Read the model definition and answer for the solid it produces. Units are mm, in the model's axes. Face numbers are marked on the shaded views. A direction names the side the tool comes from. Coordinates: 2 decimals unless noted, no trailing zeros. Order: outer loops, then holes, each group sorted by start corner. A loop starts at its lowest first (then second) coordinate and runs counter-clockwise, first axis right, second up. Notation, with made-up numbers: (-34.5, 19) -> (1.5, 19) arc R21 cw to (1.5, 45) -> close; hole circle Ø9 at (25.5, -4). An arc over 180 degrees is marked (long way). Use CSV: the item, a comma, the result in double quotes.
```python
from build123d import *

# Parameters (mm, degrees)
SKETCH1_R           = 2.5
BOSS_EXTRUDE1_DEPTH = 30


with BuildPart() as part:
    # Sketch1 → Boss-Extrude1 (new body)
    with BuildSketch(Plane.XY):
        with BuildLine():
            Line((-8, 4), (8, 4))
            ThreePointArc((8, 4), (8.707106781, 3.707106781), (9, 3))
            Line((9, 3), (9, 2))
            Line((9, 2), (21.5, 2))
            ThreePointArc((21.5, 2), (22.207106781, 1.707106781), (22.5, 1))
            Line((22.5, 1), (22.5, 0))
            Line((22.5, 0), (30, 0))
            Line((30, 0), (24.933748499, 30.8112495))
            ThreePointArc((24.933748499, 30.8112495), (23.236027851, 33.811577593), (20, 35))
            Line((20, 35), (15, 35))
            Line((15, 35), (15, 29))
            ThreePointArc((15, 29), (14.414213562, 27.585786438), (13, 27))
            Line((13, 27), (10, 27))
            ThreePointArc((10, 27), (0, 17), (-10, 27))
            Line((-10, 27), (-13, 27))
            ThreePointArc((-13, 27), (-14.414213562, 27.585786438), (-15, 29))
            Line((-15, 29), (-15, 35))
            Line((-15, 35), (-20, 35))
            ThreePointArc((-20, 35), (-23.236027851, 33.811577593), (-24.933748499, 30.8112495))
            Line((-24.933748499, 30.8112495), (-30, 0))
            Line((-30, 0), (-22.5, 0))
            Line((-22.5, 0), (-22.5, 1))
            ThreePointArc((-22.5, 1), (-22.207106781, 1.707106781), (-21.5, 2))
            Line((-21.5, 2), (-9, 2))
            Line((-9, 2), (-9, 3))
            ThreePointArc((-9, 3), (-8.707106781, 3.707106781), (-8, 4))
        make_face()
        with Locations((-20, 30)):
            Circle(SKETCH1_R, mode=Mode.SUBTRACT)
        with Locations((20, 30)):
            Circle(SKETCH1_R, mode=Mode.SUBTRACT)
    extrude(amount=BOSS_EXTRUDE1_DEPTH)


solid = part.part
```
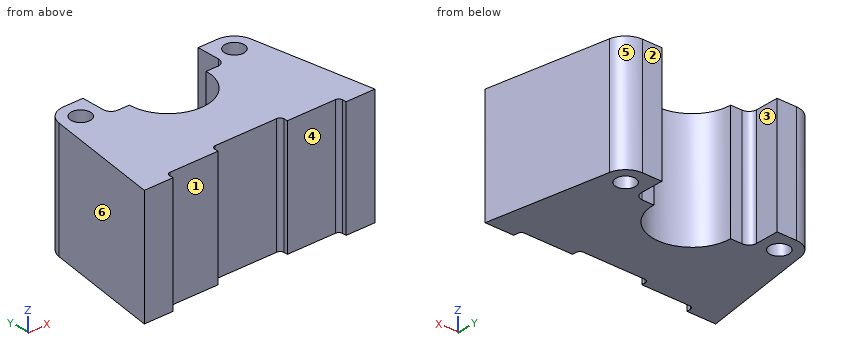
Item 1: The mould has two halves that part along X. Classify the marked faces 4, 5 and 6: +X half, -X half, draft (parallel to the pull), parting line (faces both ways), or undercut.
Return value:
face 4,"undercut"
face 5,"+X half"
face 6,"-X half"
Item 2: Each of these flat-tipped pins is pushed along its axis until it touches: P1, Ø3, axis at x = 8.5, z = 17, coming from the -Y side; P2, Ø0.9, axis at x = -11.5, z = 16, coming from the +Y side; P3, Ø1.8, axis at y = 32.5, z = 19, coming from the +X side. Where does it stop, or does it pass through?
Return value:
P1,"stops at y = 2"
P2,"stops at y = 27"
P3,"stops at x = 24.74"
Item 3: Straight lines are drawn through the part: line 1 along X through (y, z) = (32, 17.5); line 2 along X through (y, z) = (28, 7.25); line 3 along X through (y, z) = (26.5, 12.5). For each, find the intervals that lie inside material, in ascending order.
Return value:
line 1,"x = -24.58 to -21.5, -18.5 to -15, 15 to 18.5, 21.5 to 24.58"
line 2,"x = -25.4 to -21.5, -18.5 to -14.73, 14.73 to 18.5, 21.5 to 25.4"
line 3,"x = -25.64 to -9.99, 9.99 to 25.64"
Item 4: Find section C-C, the plane y = 30. Give the vertices of the cut face in (x, z).
Return value:
outline,"(-25.07, 0) -> (-22.5, 0) -> (-22.5, 30) -> (-25.07, 30) -> close; (-17.5, 0) -> (-15, 0) -> (-15, 30) -> (-17.5, 30) -> close; (15, 0) -> (17.5, 0) -> (17.5, 30) -> (15, 30) -> close; (22.5, 0) -> (25.07, 0) -> (25.07, 30) -> (22.5, 30) -> close"
Item 5: Find section D-D, the plane x = 0. Give the vertices of the cut face in (y, z).
Return value:
outline,"(4, 0) -> (17, 0) -> (17, 30) -> (4, 30) -> close"
Item 6: A tool of negligible diameter and unlimited length cuts with its end or side. For the marked faces 1, 2 and 3, from which of +Z, -Z, +X, -X, +Y, -Y can it reach the whole face along a straight path? Write none if from no direction.
Return value:
face 1,"+Z, -Z, -Y"
face 2,"+Z, -Z, +X, -X, +Y"
face 3,"+Z, -Z, +Y"
Item 7: Find section A-A, the plane z = 21.75. Give the vertices of the cut face in (x, y).
Return value:
outline,"(-30, 0) -> (-22.5, 0) -> (-22.5, 1) arc R1 cw to (-21.5, 2) -> (-9, 2) -> (-9, 3) arc R1 cw to (-8, 4) -> (8, 4) arc R1 cw to (9, 3) -> (9, 2) -> (21.5, 2) arc R1 cw to (22.5, 1) -> (22.5, 0) -> (30, 0) -> (24.93, 30.81) arc R5 ccw to (20, 35) -> (15, 35) -> (15, 29) arc R2 cw to (13, 27) -> (10, 27) arc R10 cw to (-10, 27) -> (-13, 27) arc R2 cw to (-15, 29) -> (-15, 35) -> (-20, 35) arc R5 ccw to (-24.93, 30.81) -> close; hole circle Ø5 at (-20, 30); hole circle Ø5 at (20, 30)"
Item 8: Find section B-B, the plane y = 22. Give the vertices of the cut face in (x, z).
Return value:
outline,"(-26.38, 0) -> (-8.66, 0) -> (-8.66, 30) -> (-26.38, 30) -> close; (8.66, 0) -> (26.38, 0) -> (26.38, 30) -> (8.66, 30) -> close"
